Input: part model. Units: mm. Frame: model coordinates. Face numbers are marked on the shaded views. A direction names the side the tool comes from. Give positions to 0.01 mm unless a question says otherwise; leave off trailing zeros. Answer as a JSON object with one key per item and string values. Group by question number.
from build123d import *

# Parameters (mm, degrees)
F1_DEPTH = 40
F3_DEPTH = 250.001
F5_DEPTH = 10
F6_R     = 1


with BuildPart() as f1:
    # F0 (on Top) → F1 (new body)
    with BuildSketch(Plane.XY):
        with BuildLine():
            Line((-125, 40), (-125, 0))
            Line((-125, 0), (125, 0))
            Line((125, 0), (125, 40))
            ThreePointArc((125, 40), (0, 55.8770817241), (-125, 40))
        make_face()
    extrude(amount=F1_DEPTH)

    # F2 (on face) → F3 (cut, through all)
    with BuildSketch(Plane.YZ.offset(125)):
        Polygon((5, 40), (10.6160445296, 19.0406364781), (34.7641901868, 25.5111126057), (30.8819045103, 40), align=None)
    extrude(amount=-F3_DEPTH, mode=Mode.SUBTRACT)

    # F4 (on face) → F5 (cut)
    with BuildSketch(Plane(origin=(0, 0, 0), x_dir=(1, 0, 0), z_dir=(0, 0, -1))):
        with BuildLine():
            ThreePointArc((-125, -29.6650089658), (0, -45.8770817241), (125, -29.6650089658))
            Line((125, -29.6650089658), (125, -10))
            Line((125, -10), (-125, -10))
            Line((-125, -10), (-125, -29.6650089658))
        make_face()
    extrude(amount=-F5_DEPTH, mode=Mode.SUBTRACT)

    # F6
    f6_edges = [f1.edges().sort_by_distance(p)[0] for p in [
        (0, 55.877082, 40),
        (0, 30.881905, 40),
        (-125, 35.440952, 40),
        (-125, 34.832504, 0),
        (-125, 29.665009, 5),
        (-125, 19.832504, 10),
        (-125, 10, 5),
        (-125, 5, 0),
        (-125, 0, 20),
        (-125, 2.5, 40),
        (-125, 7.808022, 29.520318),
        (-125, 22.690117, 22.275875),
        (-125, 32.823047, 32.755556),
        (-125, 40, 20),
        (125, 22.690117, 22.275875),
        (0, 34.76419, 25.511113),
        (0, 10.616045, 19.040636),
        (125, 2.5, 40),
        (0, 0, 40),
        (0, 5, 40),
        (0, 45.877082, 10),
        (125, 19.832504, 10),
        (0, 10, 10),
        (125, 29.665009, 5),
        (0, 45.877082, 0),
        (125, 34.832504, 0),
        (0, 55.877082, 0),
        (125, 5, 0),
        (0, 0, 0),
        (0, 10, 0),
        (125, 0, 20),
        (125, 10, 5),
        (125, 32.823047, 32.755556),
        (125, 7.808022, 29.520318),
    ]]
    fillet(f6_edges, radius=F6_R)


solid = f1.part
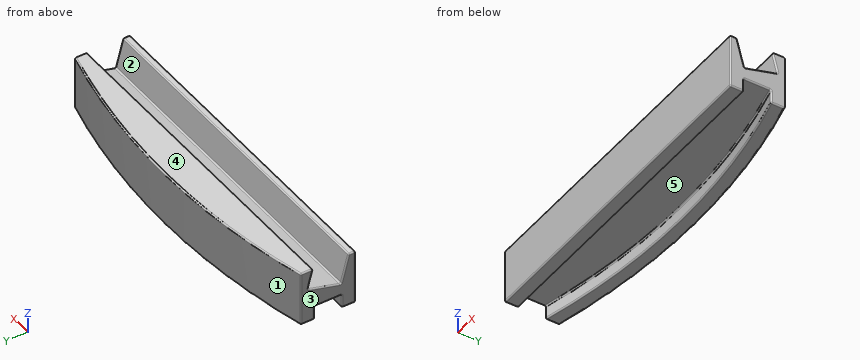
1) Reachability of the marked faces 4 and 5 from +Z, -Z, +X, -X, +Y, -Y: full face, straight path, thin tool, end or side. Return the list, or none.
2) Pin query (flat end, axial travel): P1, Ø3, axis at x = 39.5, z = 35, coming from the +Y side; P2, Ø1.5, axis at x = 79, y = 16.5, coming from the +Z side; P3, Ø1, axis at x = -75, y = 25, coming from the +Z side. Return the tip coordinate at first contact, or that it passes through.
3) Line query: line 1 along Y through (x, z) = (31.5, 7); line 2 along Z through (x, y) = (41, 40.5); line 3 along X through (y, z) = (34.5, 30). Output: solid intervals per line, ascending. Write a range as from..to.
4) Mould query, pull axis Y, two halves, no side actions, for the marked faces 1, 2 and 3. Classes: +Y half, -Y half, draft (parallel to the pull), parting line (faces both ways), or undercut.
Filled in:
{
 "1": {"face 4": "+Z, +X, -X, +Y, -Y", "face 5": "-Z"},
 "2": {"P1": "stops at y = 54.43", "P2": "stops at z = 20.82", "P3": "stops at z = 23.03"},
 "3": {"line 1": "y = 0..10, 44.86..54.88", "line 2": "z = 10..40", "line 3": "x = -125..125"},
 "4": {"face 1": "+Y half", "face 2": "undercut", "face 3": "draft"}
}
